```python
from build123d import *

# Parameters (mm, degrees)
BOSS_EXTRU_1_DEPTH           = 11
BOSS_EXTRU_1_DEPTH_BACK      = 11
ESQUISSE1_R                  = 82.5
ESQUISSE1_R_2                = 40
ESQUISSE2_R                  = 2.75
ENL_V_MAT_EXTRU_1_DEPTH      = 119.728682297
ESQUISSE4_R                  = 4.75
ENL_V_MAT_EXTRU_3_DEPTH      = 5.4
ESQUISSE5_R                  = 4.75
ENL_V_MAT_EXTRU_4_DEPTH      = 5.4
R_P_TITION_CIRCULAIRE1_COUNT = 10
ENL_V_START                  = -3
ESQUISSE3_R                  = 63.75
ESQUISSE3_R_2                = 58.75
ENL_V_MAT_EXTRU_2_DEPTH      = 122.728682297
D_GAGEMENT_M51_AT_2_COUNT    = 2
D_GAGEMENT_M51_AT_2_PITCH    = 96.989005831
D_GAGEMENT_M51_AT_3_COUNT    = 2
D_GAGEMENT_M51_AT_3_PITCH    = 92.242026005
D_GAGEMENT_M51_AT_4_COUNT    = 2
D_GAGEMENT_M51_AT_4_PITCH    = 92.242026005
D_GAGEMENT_M51_AT_5_COUNT    = 2
D_GAGEMENT_M51_AT_5_PITCH    = 57.008707262
D_GAGEMENT_M51_AT_6_COUNT    = 2
D_GAGEMENT_M51_AT_6_PITCH    = 29.971251069
D_GAGEMENT_M51_AT_7_COUNT    = 2
D_GAGEMENT_M51_AT_7_PITCH    = 57.008707262
D_GAGEMENT_M51_AT_8_COUNT    = 2
D_GAGEMENT_M51_AT_8_PITCH    = 78.465753985
D_GAGEMENT_M51_AT_9_COUNT    = 2
D_GAGEMENT_M51_AT_9_PITCH    = 29.971251069
D_GAGEMENT_M51_AT_10_COUNT   = 2
D_GAGEMENT_M51_AT_10_PITCH   = 78.465753985


with BuildPart() as part:
    # Esquisse1 → Boss.-Extru.1 (new, two sides: drawn at the far end of the back side and taken through both)
    with BuildSketch(Plane(origin=(0, 0, 0), x_dir=(1, 0, 0), z_dir=(0, 1, 0)).offset(-BOSS_EXTRU_1_DEPTH_BACK)):
        with Locations(Location((0, 0, 0), (0, 0, 270))):
            Circle(ESQUISSE1_R)
        with Locations(Location((0, 0, 0), (0, 0, 270))):
            Circle(ESQUISSE1_R_2, mode=Mode.SUBTRACT)
    extrude(amount=BOSS_EXTRU_1_DEPTH + BOSS_EXTRU_1_DEPTH_BACK)

    # Esquisse2 → Enl_v. mat.-Extru.1 (cut, symmetric)
    with BuildSketch(Plane(origin=(0, 11, 0), x_dir=(1, 0, 0), z_dir=(0, 1, 0))):
        with Locations(Location((73.541719779, 0, 0), (0, 0, 270))):
            Circle(ESQUISSE2_R)
        with Locations(Location((48.494502916, 0, 0), (0, 0, 270))):
            Circle(ESQUISSE2_R)
    enl_v_mat_extru_1 = extrude(amount=ENL_V_MAT_EXTRU_1_DEPTH, both=True, mode=Mode.SUBTRACT)

    # Esquisse4 → Enl_v. mat.-Extru.3 (cut)
    with BuildSketch(Plane(origin=(0, 11, 0), x_dir=(1, 0, 0), z_dir=(0, 1, 0))):
        with Locations(Location((73.541719779, 0, 0), (0, 0, 270))):
            Circle(ESQUISSE4_R)
    enl_v_mat_extru_3 = extrude(amount=-ENL_V_MAT_EXTRU_3_DEPTH, mode=Mode.SUBTRACT)

    # Esquisse5 → Enl_v. mat.-Extru.4 (cut)
    with BuildSketch(Plane.XZ.offset(11)):
        with Locations(Location((48.494502916, 0, 0), (0, 0, 270))):
            Circle(ESQUISSE5_R)
    enl_v_mat_extru_4 = extrude(amount=-ENL_V_MAT_EXTRU_4_DEPTH, mode=Mode.SUBTRACT)

    # R_p_tition circulaire1: Enl_v. mat.-Extru.1, Enl_v. mat.-Extru.3, Enl_v. mat.-Extru.4 ×10 about axis
    r_p_tition_circulaire1_axis = Axis((0, 0, 0), (0, 1, 0))
    add([enl_v_mat_extru_1.rotate(r_p_tition_circulaire1_axis, i * 360 / R_P_TITION_CIRCULAIRE1_COUNT) for i in range(1, R_P_TITION_CIRCULAIRE1_COUNT)], mode=Mode.SUBTRACT)
    add([enl_v_mat_extru_3.rotate(r_p_tition_circulaire1_axis, i * 360 / R_P_TITION_CIRCULAIRE1_COUNT) for i in range(1, R_P_TITION_CIRCULAIRE1_COUNT)], mode=Mode.SUBTRACT)
    add([enl_v_mat_extru_4.rotate(r_p_tition_circulaire1_axis, i * 360 / R_P_TITION_CIRCULAIRE1_COUNT) for i in range(1, R_P_TITION_CIRCULAIRE1_COUNT)], mode=Mode.SUBTRACT)

    # Esquisse3 → Enl_v. mat.-Extru.2 (cut)
    with BuildSketch(Plane(origin=(0, 11, 0), x_dir=(1, 0, 0), z_dir=(0, 1, 0)).offset(ENL_V_START)):
        with Locations(Location((0, 0, 0), (0, 0, 90))):
            Circle(ESQUISSE3_R)
        with Locations(Location((0, 0, 0), (0, 0, 90))):
            Circle(ESQUISSE3_R_2, mode=Mode.SUBTRACT)
    enl_v_mat_extru_2 = extrude(amount=ENL_V_MAT_EXTRU_2_DEPTH, mode=Mode.SUBTRACT)

    # Sym_trie1: Enl_v. mat.-Extru.2 across plane
    add(enl_v_mat_extru_2.mirror(Plane.ZX), mode=Mode.SUBTRACT)

    # Esquisse6 → D_gagement M51 (revolve, cut)
    with BuildSketch(Plane(origin=(-48.494502916, -5.6, 0), x_dir=(0, 0, -1), z_dir=(1, 0, 0))):
        Polygon((0, 0), (0, 91.742495795), (2.9, 90), (2.9, 0), align=None)
    d_gagement_m51 = revolve(axis=Axis((-48.494502916, -11.95, 0), (0, 1, 0)), mode=Mode.SUBTRACT)

    # D_gagement M51 at 2: D_gagement M51 ×2
    with Locations(*[(i * D_GAGEMENT_M51_AT_2_PITCH, 0, 0) for i in range(1, D_GAGEMENT_M51_AT_2_COUNT)]):
        add(d_gagement_m51, mode=Mode.SUBTRACT)

    # D_gagement M51 at 3: D_gagement M51 ×2
    with Locations(*[Vector(0.9510565162951522, 0, 0.3090169943749516) * (i * D_GAGEMENT_M51_AT_3_PITCH) for i in range(1, D_GAGEMENT_M51_AT_3_COUNT)]):
        add(d_gagement_m51, mode=Mode.SUBTRACT)

    # D_gagement M51 at 4: D_gagement M51 ×2
    with Locations(*[Vector(0.9510565162951545, 0, -0.3090169943749448) * (i * D_GAGEMENT_M51_AT_4_PITCH) for i in range(1, D_GAGEMENT_M51_AT_4_COUNT)]):
        add(d_gagement_m51, mode=Mode.SUBTRACT)

    # D_gagement M51 at 5: D_gagement M51 ×2
    with Locations(*[Vector(0.5877852522924744, 0, -0.8090169943749467) * (i * D_GAGEMENT_M51_AT_5_PITCH) for i in range(1, D_GAGEMENT_M51_AT_5_COUNT)]):
        add(d_gagement_m51, mode=Mode.SUBTRACT)

    # D_gagement M51 at 6: D_gagement M51 ×2
    with Locations(*[Vector(0.3090169943749479, 0, -0.9510565162951535) * (i * D_GAGEMENT_M51_AT_6_PITCH) for i in range(1, D_GAGEMENT_M51_AT_6_COUNT)]):
        add(d_gagement_m51, mode=Mode.SUBTRACT)

    # D_gagement M51 at 7: D_gagement M51 ×2
    with Locations(*[Vector(0.5877852522924686, 0, 0.8090169943749508) * (i * D_GAGEMENT_M51_AT_7_PITCH) for i in range(1, D_GAGEMENT_M51_AT_7_COUNT)]):
        add(d_gagement_m51, mode=Mode.SUBTRACT)

    # D_gagement M51 at 8: D_gagement M51 ×2
    with Locations(*[Vector(0.8090169943749447, 0, 0.587785252292477) * (i * D_GAGEMENT_M51_AT_8_PITCH) for i in range(1, D_GAGEMENT_M51_AT_8_COUNT)]):
        add(d_gagement_m51, mode=Mode.SUBTRACT)

    # D_gagement M51 at 9: D_gagement M51 ×2
    with Locations(*[Vector(0.3090169943749415, 0, 0.9510565162951555) * (i * D_GAGEMENT_M51_AT_9_PITCH) for i in range(1, D_GAGEMENT_M51_AT_9_COUNT)]):
        add(d_gagement_m51, mode=Mode.SUBTRACT)

    # D_gagement M51 at 10: D_gagement M51 ×2
    with Locations(*[Vector(0.8090169943749487, 0, -0.5877852522924714) * (i * D_GAGEMENT_M51_AT_10_PITCH) for i in range(1, D_GAGEMENT_M51_AT_10_COUNT)]):
        add(d_gagement_m51, mode=Mode.SUBTRACT)


solid = part.part
```
Can you work these out from the model? Positions are in its coordinate system, mm. A direction names the side the tool comes from. Give positions to 0.01 mm unless a question says otherwise; leave off trailing zeros. Loops run counter-clockwise (first coordinate to the right, second up) from the corner with the lowest first, then second, coordinate; pieces in that order, holes last. Notation, with made-up numbers: M -23.75,22.25 L -4.75,22.25 A35 ccw -4.75,54.25 Z; hole C 87,-13.5 d11. An arc over 180 degrees is marked long. One line per item, written item: value.
(1) Which directions (+Z, -Z, +X, -X, +Y, -Y) give clear straight access to the entire face, cutting with the end or side of a thin tool? Please do faces 1 (the face through (71, 5.6, 2)), 2 (the face through (40.344, 2.584, 25.825)), 3 (the face through (-15.768, -8.338, -41.436)).
Returned:
face 1: +Y
face 2: +Y, -Y
face 3: -Y
(2) I need wall thicknesses on line 1 (X direction, y = 2, z = 0); line 2 (Z direction, x = 20.5, y = -1.75); line 3 (Z direction, x = 25, y = -7). Which ranges of each line are inside material? Lowest first, please.
Returned:
line 1: -82.5 to -76.29, -70.79 to -51.39, -45.59 to -40, 40 to 45.59, 51.39 to 70.79, 76.29 to 82.5
line 2: -79.91 to -71.56, -68.33 to -34.35, 34.35 to 68.33, 71.56 to 79.91
line 3: -78.62 to -71.49, -68.4 to -31.22, 31.22 to 68.4, 71.49 to 78.62
(3) Suppose I cut it at B-B on z = 0. Count the separate pieces of the cut face and the enclosed holes in it, plus the area to 3 significant figures.
Returned:
separate pieces: 6
enclosed holes: 0
area: 1,230 mm^2
(4) Will these pins go through, and if not, where does the flat tip stop? pin 1 (1.5 mm diameter, centred on y = -8.5, z = -63, fed in from +X); pin 2 (8 mm diameter, centred on x = -60, z = 58.5, fed in from +Y); pin 3 (8 mm diameter, centred on x = -39.5, y = 8, fed in from -Z); pin 4 (6.5 mm diameter, centred on x = -73.54, z = 0, fed in from +Y).
Returned:
pin 1: x = 54.14
pin 2: y = 11
pin 3: z = -74.47
pin 4: y = 5.6
(5) Suppose I cut it at A-A on x = 0. List the corners of the cut face in (y, z) for me.
Returned:
outline: M -11,-82.5 L 11,-82.5 L 11,-63.75 L 8,-63.75 L 8,-58.75 L 11,-58.75 L 11,-40 L -11,-40 L -11,-58.75 L -8,-58.75 L -8,-63.75 L -11,-63.75 Z; M -11,40 L 11,40 L 11,58.75 L 8,58.75 L 8,63.75 L 11,63.75 L 11,82.5 L -11,82.5 L -11,63.75 L -8,63.75 L -8,58.75 L -11,58.75 Z
